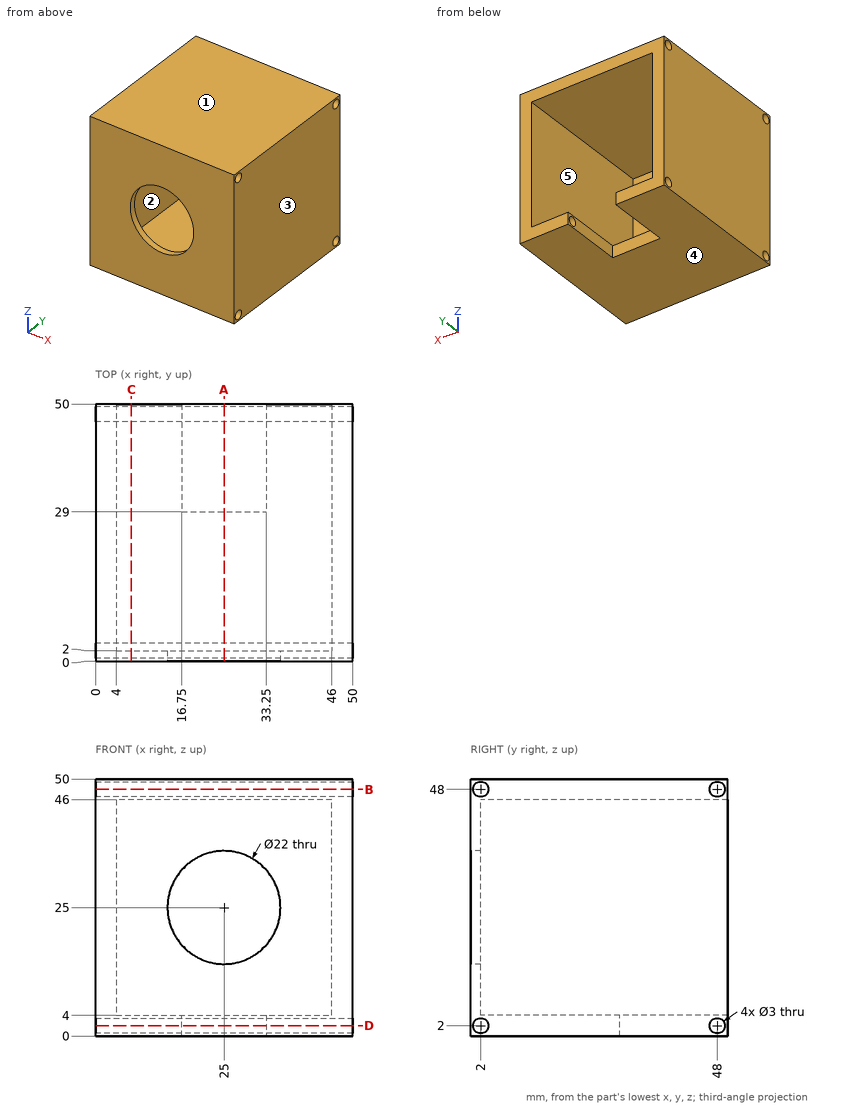
The drawing under review shows one solid part. Ordinate dimensions are in mm from its lowest x, y, z. A direction names the side the tool comes from. Coordinates: 2 decimals unless noted, no trailing zeros. Order: outer loops, then holes, each group sorted by start corner. A loop starts at its lowest first (then second) coordinate and runs counter-clockwise, first axis right, second up. Notation, with made-up numbers: M 41.25,7.25 L 70.25,7.25 A32 cw 70.25,44.25 Z; hole C 45,16.5 d10. An arc over 180 degrees is marked long. Use a Markdown table: item, result.
(1) Add section B-B (z = 48). Give the boundary of the cut face in (x, y), then the cut area to 3 significant figures.
Worked answers:
| item | result |
|---|---|
| outline | M 0,0 L 50,0 L 50,0.5 L 0,0.5 Z; M 0,3.5 L 50,3.5 L 50,46.5 L 0,46.5 Z; M 0,49.5 L 50,49.5 L 50,50 L 0,50 Z |
| area | 2,200 mm2 |
(2) Add section C-C (x = 7). Give the boundary of the cut face in (y, z).
Worked answers:
| item | result |
|---|---|
| outline | M 0,0 L 50,0 L 50,4 L 2,4 L 2,46 L 50,46 L 50,50 L 0,50 Z; hole C 2,2 d3; hole C 2,48 d3; hole C 48,2 d3; hole C 48,48 d3 |
(3) Wall thickness on probe 1 along Y at (x, z) = (29, 48); probe 2 along Z at (x, y) = (36, 36.5): over which ranges is each line inside the solid? List them lowest first.
Worked answers:
| item | result |
|---|---|
| probe 1 | y = 0 to 0.5, 3.5 to 46.5, 49.5 to 50 |
| probe 2 | z = 0 to 4, 46 to 50 |
(4) Add section A-A (x = 25). Give the boundary of the cut face in (y, z).
Worked answers:
| item | result |
|---|---|
| outline | M 0,0 L 29,0 L 29,4 L 2,4 L 2,14 L 0,14 Z; M 0,36 L 2,36 L 2,46 L 50,46 L 50,50 L 0,50 Z; hole C 2,2 d3; hole C 2,48 d3; hole C 48,48 d3 |
(5) Draft analysis for pull direction Z (two halves, no side actions). For the marked faces 1, 2 and 3, state which applies: released by +Z, released by -Z, zero draft, split by the parting line, or undercut.
Worked answers:
| item | result |
|---|---|
| face 1 | released by +Z |
| face 2 | undercut |
| face 3 | zero draft |
(6) For the marked faces 4 and 5, list the 3-axis set-ups (+Z, -Z, +X, -X, +Y, -Y) from which the entire face can be reached by the end or side of a thin tool; tool diameter is ignored.
Worked answers:
| item | result |
|---|---|
| face 4 | -Z, +X, -X, +Y, -Y |
| face 5 | +Y |
(7) For P1, Ø4.5, axis at x = 25.5, z = 1, coming from the +Y side; P2, Ø8, axis at x = 41, z = 15.5, coming from the +Y side; P3, Ø1.8, axis at y = 2, z = 2, coming from the +X side, all flat-tipped, find the tip position at first contact; note any pin that passes through.
Worked answers:
| item | result |
|---|---|
| P1 | stops at y = 29 |
| P2 | stops at y = 2 |
| P3 | passes through |
(8) Add section D-D (z = 2). Give the boundary of the cut face in (x, y), then the cut area to 3 significant figures.
Worked answers:
| item | result |
|---|---|
| outline | M 0,0 L 50,0 L 50,0.5 L 0,0.5 Z; M 0,3.5 L 50,3.5 L 50,46.5 L 33.25,46.5 L 33.25,29 L 16.75,29 L 16.75,46.5 L 0,46.5 Z; M 0,49.5 L 16.75,49.5 L 16.75,50 L 0,50 Z; M 33.25,49.5 L 50,49.5 L 50,50 L 33.25,50 Z |
| area | 1,900 mm2 |
